```python
from build123d import *

# Parameters (mm, degrees)
BOSS_EXTRUDE3_DEPTH = 50
SKETCH4_W           = 14.85
SKETCH4_H           = 5
BOSS_EXTRUDE4_DEPTH = 26
SKETCH6_W           = 26
SKETCH6_H           = 5
BOSS_EXTRUDE5_DEPTH = 3
SKETCH7_W           = 26
SKETCH7_H           = 5
BOSS_EXTRUDE6_DEPTH = 3
BOSS_EXTRUDE7_DEPTH = 45
CUT_EXTRUDE1_START  = -5
CUT_EXTRUDE1_DEPTH  = 5


with BuildPart() as part:
    # Sketch1 → Boss-Extrude3 (new body)
    with BuildSketch(Plane(origin=(0, 0, 0), x_dir=(1, 0, 0), z_dir=(0, 1, 0))):
        with BuildLine():
            Line((5.249679656, 8.303679656), (10.918893219, 13.972893219))
            ThreePointArc((10.918893219, 13.972893219), (11.13566597, 15.062683432), (10.211786438, 15.68))
            Line((10.211786438, 15.68), (6.065, 15.68))
            ThreePointArc((6.065, 15.68), (4.650786438, 16.265786438), (4.065, 17.68))
            Line((4.065, 17.68), (4.065, 18))
            ThreePointArc((4.065, 18), (4.650786438, 19.414213562), (6.065, 20))
            Line((6.065, 20), (18, 20))
            ThreePointArc((18, 20), (19.414213562, 19.414213562), (20, 18))
            Line((20, 18), (20, 6.065))
            ThreePointArc((20, 6.065), (19.414213562, 4.650786438), (18, 4.065))
            Line((18, 4.065), (17.68, 4.065))
            ThreePointArc((17.68, 4.065), (16.265786438, 4.650786438), (15.68, 6.065))
            Line((15.68, 6.065), (15.68, 10.211786438))
            ThreePointArc((15.68, 10.211786438), (15.062683432, 11.13566597), (13.972893219, 10.918893219))
            Line((13.972893219, 10.918893219), (8.303679656, 5.249679656))
            ThreePointArc((8.303679656, 5.249679656), (7.653361402, 4.27640961), (7.425, 3.128359313))
            Line((7.425, 3.128359313), (7.425, -3.128359313))
            ThreePointArc((7.425, -3.128359313), (7.653361402, -4.27640961), (8.303679656, -5.249679656))
            Line((8.303679656, -5.249679656), (13.972893219, -10.918893219))
            ThreePointArc((13.972893219, -10.918893219), (15.062683432, -11.13566597), (15.68, -10.211786438))
            Line((15.68, -10.211786438), (15.68, -6.065))
            ThreePointArc((15.68, -6.065), (16.265786438, -4.650786438), (17.68, -4.065))
            Line((17.68, -4.065), (18, -4.065))
            ThreePointArc((18, -4.065), (19.414213562, -4.650786438), (20, -6.065))
            Line((20, -6.065), (20, -18))
            ThreePointArc((20, -18), (19.414213562, -19.414213562), (18, -20))
            Line((18, -20), (6.065, -20))
            ThreePointArc((6.065, -20), (4.650786438, -19.414213562), (4.065, -18))
            Line((4.065, -18), (4.065, -17.68))
            ThreePointArc((4.065, -17.68), (4.650786438, -16.265786438), (6.065, -15.68))
            Line((6.065, -15.68), (10.211786438, -15.68))
            ThreePointArc((10.211786438, -15.68), (11.13566597, -15.062683432), (10.918893219, -13.972893219))
            Line((10.918893219, -13.972893219), (5.249679656, -8.303679656))
            ThreePointArc((5.249679656, -8.303679656), (4.27640961, -7.653361402), (3.128359313, -7.425))
            Line((3.128359313, -7.425), (0, -7.425))
            Line((0, -7.425), (0, 7.425))
            Line((0, 7.425), (3.128359313, 7.425))
            ThreePointArc((3.128359313, 7.425), (4.27640961, 7.653361402), (5.249679656, 8.303679656))
        make_face()
    boss_extrude3 = extrude(amount=BOSS_EXTRUDE3_DEPTH)

    # Sketch4 → Boss-Extrude4 (add)
    with BuildSketch(Plane.ZY):
        with Locations((0, 2.5)):
            Rectangle(SKETCH4_W, SKETCH4_H)
    extrude(amount=BOSS_EXTRUDE4_DEPTH)

    # Mirror2: Boss-Extrude3 across plane
    add(boss_extrude3.mirror(Plane.ZY.offset(13)))

    # Sketch6 → Boss-Extrude5 (add)
    with BuildSketch(Plane.XY.offset(7.425)):
        with Locations((-13, 2.5)):
            Rectangle(SKETCH6_W, SKETCH6_H)
    extrude(amount=BOSS_EXTRUDE5_DEPTH)

    # Sketch7 → Boss-Extrude6 (add)
    with BuildSketch(Plane(origin=(0, 0, -7.425), x_dir=(-1, 0, 0), z_dir=(0, 0, -1))):
        with Locations((13, 2.5)):
            Rectangle(SKETCH7_W, SKETCH7_H)
    extrude(amount=BOSS_EXTRUDE6_DEPTH)

    # Sketch8 → Boss-Extrude7 (add)
    with BuildSketch(Plane(origin=(0, 5, 0), x_dir=(1, 0, 0), z_dir=(0, 1, 0))):
        with BuildLine():
            Line((-23, 10.425), (-3, 10.425))
            ThreePointArc((-3, 10.425), (-0.878679656, 9.546320344), (0, 7.425))
            Line((0, 7.425), (0, 6))
            Line((0, 6), (-26, 6))
            Line((-26, 6), (-26, 7.425))
            ThreePointArc((-26, 7.425), (-25.121320344, 9.546320344), (-23, 10.425))
        make_face()
        with BuildLine():
            Line((0, -7.425), (0, -6))
            Line((0, -6), (-26, -6))
            Line((-26, -6), (-26, -7.425))
            ThreePointArc((-26, -7.425), (-25.121320344, -9.546320344), (-23, -10.425))
            Line((-23, -10.425), (-3, -10.425))
            ThreePointArc((-3, -10.425), (-0.878679656, -9.546320344), (0, -7.425))
        make_face()
    extrude(amount=BOSS_EXTRUDE7_DEPTH)

    # Sketch9 → Cut-Extrude1 (cut)
    with BuildSketch(Plane(origin=(0, 5, 0), x_dir=(1, 0, 0), z_dir=(0, 1, 0)).offset(CUT_EXTRUDE1_START)):
        with BuildLine():
            Line((-3, -10.425), (0, -10.425))
            Line((0, -10.425), (0, -7.425))
            ThreePointArc((0, -7.425), (-0.878679656, -9.546320344), (-3, -10.425))
        make_face()
        with BuildLine():
            Line((-26, -10.425), (-26, -7.425))
            ThreePointArc((-26, -7.425), (-25.121320344, -9.546320344), (-23, -10.425))
            Line((-23, -10.425), (-26, -10.425))
        make_face()
        with BuildLine():
            Line((0, 10.425), (0, 7.425))
            ThreePointArc((0, 7.425), (-0.878679656, 9.546320344), (-3, 10.425))
            Line((-3, 10.425), (0, 10.425))
        make_face()
        with BuildLine():
            Line((-23, 10.425), (-26, 10.425))
            Line((-26, 10.425), (-26, 7.425))
            ThreePointArc((-26, 7.425), (-25.121320344, 9.546320344), (-23, 10.425))
        make_face()
    extrude(amount=CUT_EXTRUDE1_DEPTH, mode=Mode.SUBTRACT)


solid = part.part
```
Build history of the part. All positions in model axes, mm. A direction names the side the tool comes from. Give positions to 0.01 mm unless a question says otherwise; leave off trailing zeros. Loops run counter-clockwise (first coordinate to the right, second up) from the corner with the lowest first, then second, coordinate; pieces in that order, holes last. Notation, with made-up numbers: (-38.75, -5.5) -> (-32.75, -5.5) arc R19 ccw to (-32.75, 7.5) -> close; hole circle Ø2 at (-23, 79.25). An arc over 180 degrees is marked (long way). One line per question, with ' | ' between items. Start each with the question number.
1) Cut at D-D (z = 0). Give the cut face in (x, y) (3 decimals), plus the area to 4 significant figures.
2) 3-axis set-ups, long thin cutter, end or side, ignore diameter. For faces 1 (the cylindrical face through (19.399, 24.65, 4.635)), 2 (the cylindrical face through (-25.145, 24.65, 9.523)), 3 (the cylindrical face through (11.13, 24.65, 15.08)): which of +Z, -Z, +X, -X, +Y, -Y reach the whole face in a straight line?
3) Cut at A-A (z = -13). Give the cut face in (x, y), plus the area to 3 significant figures.
4) Cut at B-B (x = -11.5). Give the cut face in (y, z) (3 decimals), plus the area to 4 significant figures.
5) Probe L1, parallel to Z at x = -3, y = 19.5 (3 decimals); L2, parallel to X at y = 40, z = 17.5; L3, parallel to X at y = 45, z = 1 (3 decimals). List the from-to ranges inside material, lowest first.
6) Cut at C-C (x = 13). Give the cut face in (y, z).
7) Pin check, flat tips, straight feed: pin 1 (8 mm diameter, centred on x = -15, y = 27, fed in from +Z) (3 decimals); pin 2 (5 mm diameter, centred on x = -0.5, y = 36, fed in from -Z) (3 decimals); pin 3 (1.6 mm diameter, centred on x = 2, y = 28, fed in from -Z) (3 decimals). Stop position of each tip, or through.
8) Two-plate mould, pull along X, no slides. Class faces 4 (the flat face through (7.425, 25, 0)), 5 (the flat face through (-34, 25, -15.68)), 6 (the cylindrical face through (-45.4, 24.65, -19.43)): released by +X, released by -X, zero draft, split by the parting line, or undercut.
Return value:
1) outline: (-33.425, 0) -> (7.425, 0) -> (7.425, 50) -> (0, 50) -> (0, 5) -> (-26, 5) -> (-26, 50) -> (-33.425, 50) -> close | area: 872.5 mm^2
2) face 1: +X, +Y, -Y | face 2: +Z, +Y, -Y | face 3: +Y, -Y
3) outline: (-46, 0) -> (-35.95, 0) -> (-35.95, 50) -> (-46, 50) -> close; (9.95, 0) -> (20, 0) -> (20, 50) -> (9.95, 50) -> close | area: 1,010 mm^2
4) outline: (0, -10.425) -> (50, -10.425) -> (50, -6) -> (5, -6) -> (5, 6) -> (50, 6) -> (50, 10.425) -> (0, 10.425) -> close | area: 502.5 mm^2
5) L1: -10.425 to -6, 6 to 10.425 | L2: -46 to -30.07, 4.07 to 20 | L3: -33.425 to -26, 0 to 7.425
6) outline: (0, -20) -> (50, -20) -> (50, -9.95) -> (0, -9.95) -> close; (0, 9.95) -> (50, 9.95) -> (50, 20) -> (0, 20) -> close
7) pin 1: z = 10.425 | pin 2: z = -10.425 | pin 3: z = -7.425
8) face 4: released by +X | face 5: undercut | face 6: released by -X
